Check sheet for the modelled part. Datum: model origin and axes. Units: mm. A direction names the side the tool comes from. Give positions to 0.01 mm unless a question says otherwise; leave off trailing zeros. Order: outer loops, then holes, each group sorted by start corner. A loop starts at its lowest first (then second) coordinate and runs counter-clockwise, first axis right, second up. Notation, with made-up numbers: M 4.25,28 L 30.25,28 A34 ccw 30.25,66 Z; hole C 29.5,-5 d10. An arc over 180 degrees is marked long. Answer in a Markdown table with one row per item. Add a question column.
from build123d import *

# Parameters (mm, degrees)
SKETCH_R        = 2
PAD_DEPTH       = 19.8
SKETCH001_W     = 89
SKETCH001_H     = 8
POCKET_DEPTH    = 16
SKETCH002_R     = 2
POCKET001_DEPTH = 115.001
CHAMFER_SIZE    = 2
CHAMFER001_SIZE = 1


with BuildPart() as part:
    # Sketch → Pad (new body)
    with BuildSketch(Plane.XY):
        Polygon((0, 9.9), (109, 9.9), (109, 25), (115, 25), (115, -25), (109, -25), (109, -9.9), (0, -9.9), align=None)
        with Locations((5, 0)):
            Circle(SKETCH_R, mode=Mode.SUBTRACT)
        with Locations((15, 0)):
            Circle(SKETCH_R, mode=Mode.SUBTRACT)
    extrude(amount=PAD_DEPTH)

    # Sketch001 (on Face12 of Pad) → Pocket (cut)
    with BuildSketch(Plane.XY.offset(19.8)):
        with Locations((64.5, -5.9)):
            Rectangle(SKETCH001_W, SKETCH001_H)
        with Locations((64.5, 5.9)):
            Rectangle(SKETCH001_W, SKETCH001_H)
    extrude(amount=-POCKET_DEPTH, mode=Mode.SUBTRACT)

    # Sketch002 (on Face9 of Pocket) → Pocket001 (cut, through all)
    with BuildSketch(Plane.YZ.offset(115)):
        with Locations((-17.5, 9.9)):
            Circle(SKETCH002_R)
        with Locations((17.5, 9.9)):
            Circle(SKETCH002_R)
    extrude(amount=-POCKET001_DEPTH, mode=Mode.SUBTRACT)

    # Chamfer
    chamfer_edges = [part.edges().sort_by_distance(p)[0] for p in [
        (109, -19.5, 9.9),
        (109, 15.5, 9.9),
    ]]
    chamfer(chamfer_edges, length=CHAMFER_SIZE)

    # Chamfer001
    chamfer001_edges = [part.edges().sort_by_distance(p)[0] for p in [
        (0, -9.9, 9.9),
        (0, 9.9, 9.9),
        (0, 0, 19.8),
        (0, 0, 0),
        (54.5, 9.9, 0),
        (54.5, -9.9, 0),
        (64.5, 9.9, 3.8),
        (64.5, -9.9, 3.8),
        (20, -9.9, 11.8),
        (10, -9.9, 19.8),
        (20, -5.9, 19.8),
        (20, 5.9, 19.8),
        (10, 9.9, 19.8),
        (20, 9.9, 11.8),
        (64.5, -1.9, 19.8),
        (64.5, 1.9, 19.8),
        (109, -17.45, 0),
        (109, 17.45, 0),
        (109, -17.45, 19.8),
        (109, 17.45, 19.8),
        (109, -25, 9.9),
        (109, 25, 9.9),
    ]]
    chamfer(chamfer001_edges, length=CHAMFER001_SIZE)


solid = part.part
Q1. Draft check along Y on faces 5 (the flat face through (64, 1.9, 11)), 6 (the flat face through (64, 5, 3.8)), 7 (the cylindrical face through (13.4, -1.2, 9.8)). Enter one of: pulls with the +Y half, pulls with the -Y half, needs draft (parallel to the pull), parting line crosses it, or undercut.
Q2. Tool access check on faces 1 (the flat face through (30.7, 9.9, 2.6)), 2 (the flat face through (109, -13, 10)), 3 (the flat face through (20, 5, 11)), 4 (the flat face through (31.3, -9.9, 2.6)). Record the directions out of +Z, -Z, +X, -X, +Y, -Y that give a thin tool (end or side, any length) a straight path to the whole face; none if there is none.
Q3. Thickness scan on probe 1 along Y at (x, z) = (5, 13); probe 2 along Z at (x, y) = (112.4, -17.5); probe 3 along X at (y, z) = (4.5, 4.25). Record the ranges inside material, lowest first.
Q4. Cross-section at D-D (y = -6). Record the boundary of the cut face in (x, z).
Q5. Cross-section at C-C (x = 5). Record the boundary of the cut face in (y, z), and give its area (3 significant figures).
Q6. Cross-section at B-B (y = 17.5). Record the boundary of the cut face in (x, z).
Q7. Cross-section at A-A (z = 9.9). State how many separate pieces and enclosed holes the cut face has, and give its area (3 significant figures).
Q8. Go/stop test with flat-tipped pins: pin 1 (1.5 mm diameter, centred on x = 38, y = 8.5, fed in from +Z); pin 2 (6 mm diameter, centred on x = 85, z = 13.5, fed in from +Y); pin 3 (10 mm diameter, centred on x = 51, y = -16, fed in from -Z); pin 4 (9 mm diameter, centred on x = 38.5, z = 9, fed in from -Y). Record where each tip stops, or that it passes through.
Values follow:
| question | item | result |
|---|---|---|
| 1 | face 5 | pulls with the +Y half |
| 1 | face 6 | needs draft |
| 1 | face 7 | undercut |
| 2 | face 1 | +Z, -Z, -X, +Y |
| 2 | face 2 | +Z, -Y |
| 2 | face 3 | +Z, +Y |
| 2 | face 4 | +Z, -Z, -X, -Y |
| 3 | probe 1 | -9.9 to -2, 2 to 9.9 |
| 3 | probe 2 | 0 to 7.9, 11.9 to 19.8 |
| 3 | probe 3 | 0 to 20, 109 to 115 |
| 4 | outline | M 0,1 L 1,0 L 115,0 L 115,19.8 L 110,19.8 L 109,18.8 L 109,3.8 L 20,3.8 L 20,18.8 L 19,19.8 L 1,19.8 L 0,18.8 Z |
| 5 | outline | M -9.9,1 L -8.9,0 L -2,0 L -2,19.8 L -8.9,19.8 L -9.9,18.8 Z; M 2,0 L 8.9,0 L 9.9,1 L 9.9,18.8 L 8.9,19.8 L 2,19.8 Z |
| 5 | area | 311 mm² |
| 6 | outline | M 109,1 L 110,0 L 115,0 L 115,7.9 L 111,7.9 L 109,5.9 Z; M 109,13.9 L 111,11.9 L 115,11.9 L 115,19.8 L 110,19.8 L 109,18.8 Z |
| 7 | separate pieces | 3 |
| 7 | enclosed holes | 2 |
| 7 | area | 950 mm² |
| 8 | pin 1 | z = 3.8 |
| 8 | pin 2 | y = 1.9 |
| 8 | pin 3 | through |
| 8 | pin 4 | y = -1.9 |
